Here's how the part is built. I have some questions about the finished solid (model axes, mm). Face numbers are marked on the shaded views. A direction names the side the tool comes from. Give positions to 0.01 mm unless a question says otherwise; leave off trailing zeros. Write each loop counter-clockwise with the first axis right and the second up, starting at its lowest first coordinate (ties: lowest second). Pieces come first, ordered by that corner, then holes. Notation, with made-up numbers: (4, 30.25) - (8, 30.25) arc R16 ccw to (8, 35.25) - close; hole circle Ø10 at (-9, 46). An arc over 180 degrees is marked (long way). Use a Markdown table: item, result.
Autodesk Fusion 360 part; units mm, degrees
sketch "Sketch1" plane through (0, 0, 0) normal (0, 1, 0) x (1, 0, 0)
  line L0 (0, 0) -> (38.8, 0)
  line L1 (38.8, 0) -> (38.8, 55)
  line L2 (38.8, 55) -> (0, 55)
  line L3 (0, 55) -> (0, 0)
  line L4 (-10, 65) -> (48.8, 65)
  line L5 (48.8, 65) -> (48.8, -10)
  line L6 (48.8, -10) -> (-10, -10)
  line L7 (-10, -10) -> (-10, 65)
  circle A0 centre (-5, 60) radius 1.45
  circle A1 centre (43.8, 60) radius 1.45
  circle A2 centre (-5, -5) radius 1.45
  circle A3 centre (43.8, -5) radius 1.45
  dimension "d1" = 55
  dimension "d2" = 38.8
  dimension "d3" = 10
  dimension "d4" = 10
  dimension "d5" = 10
  dimension "d6" = 10
  dimension "d7" = 2.9
  dimension "d8" = 2.9
  dimension "d9" = 2.9
  dimension "d10" = 2.9
  dimension "d11" = 5
  dimension "d12" = 5
  dimension "d13" = 5
  dimension "d14" = 5
  dimension "d15" = 5
  dimension "d16" = 5
  dimension "d17" = 5
  dimension "d18" = 5
extrude "Extrude1" add sketch "Sketch1" along normal blind 3 contours L0 L1 L2 L3
extrude "Extrude2" add sketch "Sketch1" along normal blind 13
sketch "Sketch2" plane through (48.8, 0, 0) normal (1, 0, 0) x (0, 0, -1)
  line L0 (-10, 0) -> (65, 0)
  line L1 (65, 0) -> (65, 13)
  line L2 (65, 13) -> (-10, 13)
  line L3 (-10, 13) -> (-10, 0)
  line L4 (-10, 13) -> (0, 13)
  line L5 (0, 0) -> (-10, 0)
  line L6 (-10, 0) -> (-10, 13)
  line L7 (0, 13) -> (6.675, 13)
  line L8 (6.675, 13) -> (6.675, 0)
  line L9 (6.675, 0) -> (0, 0)
  line L10 (6.675, 13) -> (15.675, 13)
  line L11 (15.675, 13) -> (15.675, 3)
  line L12 (15.675, 3) -> (6.675, 3)
  line L13 (6.675, 3) -> (6.675, 13)
  line L14 (65, 0) -> (-10, 0)
  dimension "d23" = 6.675
  dimension "d24" = 9
  dimension "d25" = 3
extrude "Extrude3" cut sketch "Sketch2" against normal blind 10 contours L2 L8 L10 L11 L12 L13
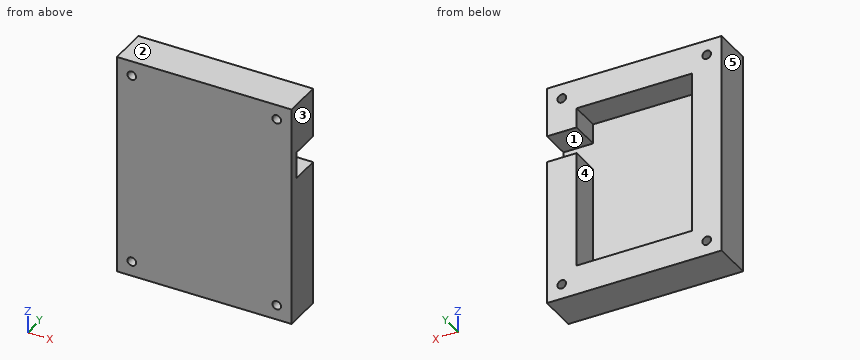
Item 1: Will these pins go through, and if not, where does the flat tip stop? pin 1 Ø1.7 at (x, z) = (43.8, 5) entering from -Y; pin 2 Ø1.5 at (x, z) = (2.5, -24.5) entering from +Y.
Values:
| item | result |
|---|---|
| pin 1 | passes through |
| pin 2 | stops at y = 3 |
Item 2: I need wall thicknesses on line 1 along X through (y, z) = (4, 5); line 2 along Z through (x, y) = (-5, 4.75); line 3 along Z through (x, y) = (43.8, 6.25) (3 decimals). Which ranges of each line are inside material? Lowest first, please. Write a range as [from, to].
Values:
| item | result |
|---|---|
| line 1 | x = [-10, -6.45], [-3.55, 42.35], [45.25, 48.8] |
| line 2 | z = [-65, -61.45], [-58.55, 3.55], [6.45, 10] |
| line 3 | z = [-65, -61.45], [-58.55, -15.675], [-6.675, 3.55], [6.45, 10] |
Item 3: If we section it at C-C, the plane y = 4.25: Write out the boundary of the cut face in (x, z) (3 decimals).
Values:
| item | result |
|---|---|
| outline | (-10, -65) - (48.8, -65) - (48.8, -15.675) - (38.8, -15.675) - (38.8, -55) - (0, -55) - (0, 0) - (38.8, 0) - (38.8, -6.675) - (48.8, -6.675) - (48.8, 10) - (-10, 10) - close; hole circle Ø2.9 at (-5, -60); hole circle Ø2.9 at (-5, 5); hole circle Ø2.9 at (43.8, -60); hole circle Ø2.9 at (43.8, 5) |
Item 4: If we section it at B-B, the plane z = -60: Write out the boundary of the cut face in (x, y), plus the area to 3 significant figures.
Values:
| item | result |
|---|---|
| outline | (-10, 0) - (-6.45, 0) - (-6.45, 13) - (-10, 13) - close; (-3.55, 0) - (42.35, 0) - (42.35, 13) - (-3.55, 13) - close; (45.25, 0) - (48.8, 0) - (48.8, 13) - (45.25, 13) - close |
| area | 689 mm2 |
Item 5: If we section it at D-D, the plane x = 28: Write out the boundary of the cut face in (y, z).
Values:
| item | result |
|---|---|
| outline | (0, -65) - (13, -65) - (13, -55) - (3, -55) - (3, 0) - (13, 0) - (13, 10) - (0, 10) - close |
Item 6: If we section it at A-A, the plane x = 43.8: Write out the boundary of the cut face in (y, z) (3 decimals).
Values:
| item | result |
|---|---|
| outline | (0, -65) - (13, -65) - (13, -61.45) - (0, -61.45) - close; (0, -58.55) - (13, -58.55) - (13, -15.675) - (3, -15.675) - (3, -6.675) - (13, -6.675) - (13, 3.55) - (0, 3.55) - close; (0, 6.45) - (13, 6.45) - (13, 10) - (0, 10) - close |
Item 7: For the marked faces 4 and 5, which set-ups out of +Z, -Z, +X, -X, +Y, -Y let a thin tool reach every point of the face, with its end or its side?
Values:
| item | result |
|---|---|
| face 4 | +Y |
| face 5 | +Z, -Z, -X, +Y, -Y |
Item 8: Thinking about a two-plate mould opening in Z: for the marked faces 1, 2 and 3, which applies, +Z half, -Z half, draft (parallel to the pull), parting line (faces both ways), or undercut?
Values:
| item | result |
|---|---|
| face 1 | undercut |
| face 2 | +Z half |
| face 3 | draft |
